Read the model definition and answer for the solid it produces. Units are mm, in the model's axes. Face numbers are marked on the shaded views. A direction names the side the tool comes from. Round coordinates to 2 decimals unless told otherwise and drop trailing zeros. Loops run counter-clockwise (first coordinate to the right, second up) from the corner with the lowest first, then second, coordinate; pieces in that order, holes last. Notation, with made-up numbers: M -32,-33 L 4,-33 A19 cw 4,-19 Z; hole C -6.5,55.25 d9. An arc over 180 degrees is marked long. Answer as CSV lines item,"result".
```python
from build123d import *

# Parameters (mm, degrees)
ENL_V_MAT_EXTRU_1_DEPTH = 9.89


with BuildPart() as part:
    # Esquisse1 → Révolution1 (revolve)
    with BuildSketch(Plane.XY):
        Polygon((-5.08, 36.25), (5.08, 36.25), (5.08, 28.8925), (1.905, 28.8925), (1.905, 10.16), (3.81, 10.16), (3.81, 0), (-3.81, 0), (-3.81, 10.16), (-1.905, 10.16), (-1.905, 28.8925), (-5.08, 28.8925), align=None)
    revolve(axis=Axis((-12.56603466, 0, 0), (1, 0, 0)))

    # Esquisse2 → Enlèv. mat.-Extru.1 (cut, through all)
    with BuildSketch(Plane(origin=(3.81, 0, 0), x_dir=(0, 0, -1), z_dir=(1, 0, 0))):
        Polygon((0, 7.332348419), (-6.35, 3.666174209), (-6.35, -3.666174209), (0, -7.332348419), (6.35, -3.666174209), (6.35, 3.666174209), align=None)
    extrude(amount=-ENL_V_MAT_EXTRU_1_DEPTH, mode=Mode.SUBTRACT)


solid = part.part
```
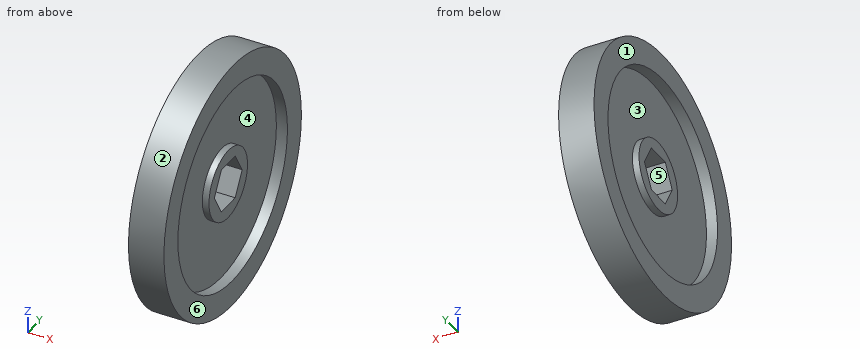
1) Determine the mould class of the marked faces 1, 2 and 3 for opening direction Y: released by +Y, released by -Y, zero draft, split by the parting line, or undercut.
Evaluation:
face 1,"zero draft"
face 2,"split by the parting line"
face 3,"undercut"
2) Each of these flat-tipped pins is pushed along its axis until it touches: P1, Ø22.5, axis at y = 2.5, z = -1, coming from the +X side; P2, Ø4, axis at x = -3, y = -14.5, coming from the +Z side; P3, Ø4, axis at x = 3, z = 9.5, coming from the +Y side. Where does it stop, or does it pass through?
Evaluation:
P1,"stops at x = 3.81"
P2,"stops at z = 34.03"
P3,"stops at y = 35.47"
3) Find section C-C, the plane z = 5.5. Give the vertices of the cut face in (x, y) (3 decimals).
Evaluation:
outline,"M -5.08,-35.83 L 5.08,-35.83 L 5.08,-28.364 L 1.905,-28.364 L 1.905,-8.543 L 3.81,-8.543 L 3.81,-4.157 L -3.81,-4.157 L -3.81,-8.543 L -1.905,-8.543 L -1.905,-28.364 L -5.08,-28.364 Z; M -5.08,28.364 L -1.905,28.364 L -1.905,8.543 L -3.81,8.543 L -3.81,4.157 L 3.81,4.157 L 3.81,8.543 L 1.905,8.543 L 1.905,28.364 L 5.08,28.364 L 5.08,35.83 L -5.08,35.83 Z"
4) Find section A-A, the plane x = -2.75. Count the separate pieces of the cut face and the enclosed holes in it, then the cut area to 3 significant figures.
Evaluation:
separate pieces,"2"
enclosed holes,"2"
area,"1,690 mm^2"
5) Find section D-D, the plane y = -16.5. Give the vertices of the cut face in (x, z) (3 decimals).
Evaluation:
outline,"M -5.08,-32.277 L 5.08,-32.277 L 5.08,-23.718 L 1.905,-23.718 L 1.905,23.718 L 5.08,23.718 L 5.08,32.277 L -5.08,32.277 L -5.08,23.718 L -1.905,23.718 L -1.905,-23.718 L -5.08,-23.718 Z"
6) A tool of negligible diameter and unlimited length cuts with its end or side. For the marked faces 4, 5 and 6, from which of +Z, -Z, +X, -X, +Y, -Y can it reach the whole face along a straight path? Write none if from no direction.
Evaluation:
face 4,"+X"
face 5,"+X, -X"
face 6,"+Z, -Z, +X, +Y, -Y"
7) Straight lines are drawn through the part: line 1 (Z direction, x = -2.9, y = 0); line 2 (Z direction, x = -1.5, y = 1); line 3 (Y direction, x = -3.5, z = 4.5). For each, find the intervals that lie inside material, in ascending order.
Evaluation:
line 1,"z = -36.25 to -28.89, -10.16 to -6.35, 6.35 to 10.16, 28.89 to 36.25"
line 2,"z = -36.24 to -6.35, 6.35 to 36.24"
line 3,"y = -35.97 to -28.54, -9.11 to -4.73, 4.73 to 9.11, 28.54 to 35.97"
